Work out the finished part from the listing and answer in its coordinate system (mm). A direction names the side the tool comes from. Give positions to 0.01 mm unless a question says otherwise; leave off trailing zeros. Loops run counter-clockwise (first coordinate to the right, second up) from the corner with the lowest first, then second, coordinate; pieces in that order, holes last. Notation, with made-up numbers: M -21.5,54 L -6.5,54 A22 cw -6.5,92 Z; hole C 55.5,-7 d5. An arc over 180 degrees is marked long. Answer in a Markdown table with one row per item. Add a question column.
from build123d import *

# Parameters (mm, degrees)
BOSS_EXTRUDE1_DEPTH = 1
CUT_EXTRUDE1_DEPTH  = 40.307328833
BOSS_EXTRUDE2_DEPTH = 10
LPATTERN1_COUNT     = 2
LPATTERN1_PITCH     = 20
CUT_EXTRUDE2_REACH  = 73.91
SKETCH4_R           = 1.75
CUT_EXTRUDE3_REACH  = 41.829
SKETCH5_W           = 10
SKETCH5_H           = 6
CHAMFER1_START      = -11.379677933
CHAMFER1_OUTLINE_W  = 13
CHAMFER1_OUTLINE_H  = 2
CHAMFER1_DEPTH      = 16.961310673


with BuildPart() as part:
    # Sketch1 → Boss-Extrude1 (new body)
    with BuildSketch(Plane.XY):
        with BuildLine():
            Line((4.5, -13.81), (34.5, -18.81))
            Line((34.5, -18.81), (34.5, 18.81))
            Line((34.5, 18.81), (-34.5, 18.81))
            Line((-34.5, 18.81), (-34.5, 14.81))
            Line((-34.5, 14.81), (-26.5, 15.18758956))
            ThreePointArc((-26.5, 15.18758956), (-6.254140463, 8.574228065), (4.5, -9.81))
            Line((4.5, -9.81), (4.5, -13.81))
        make_face()
    extrude(amount=BOSS_EXTRUDE1_DEPTH)

    # Sketch2 → Cut-Extrude1 (cut, through all)
    with BuildSketch(Plane.XY.offset(1)):
        with BuildLine():
            Line((7.75, -9.31), (29.75, -9.31))
            ThreePointArc((29.75, -9.31), (31.75, -11.31), (29.75, -13.31))
            Line((29.75, -13.31), (7.75, -13.31))
            ThreePointArc((7.75, -13.31), (5.75, -11.31), (7.75, -9.31))
        make_face()
    extrude(amount=-CUT_EXTRUDE1_DEPTH, mode=Mode.SUBTRACT)

    # Sketch3 → Boss-Extrude2 (add)
    with BuildSketch(Plane(origin=(34.5, 0, 0), x_dir=(0, 0, -1), z_dir=(1, 0, 0))):
        with BuildLine():
            Line((-1, 18.81), (-4.5, 18.81))
            ThreePointArc((-4.5, 18.81), (-7.5, 15.81), (-4.5, 12.81))
            Line((-4.5, 12.81), (-1, 12.81))
            Line((-1, 12.81), (-1, 18.81))
        make_face()
    boss_extrude2 = extrude(amount=-BOSS_EXTRUDE2_DEPTH)

    # LPattern1: Boss-Extrude2 ×2
    with Locations(*[(-i * LPATTERN1_PITCH, 0, 0) for i in range(1, LPATTERN1_COUNT)]):
        add(boss_extrude2)

    # Cut-Extrude2: up to this face of the body (flat: up to its plane)
    cut_extrude2_end = Plane(part.part.faces().sort_by_distance((4.5, 15.81, 3.966377012))[0])
    # Sketch4 → Cut-Extrude2 (cut, up to the picked face)
    with BuildSketch(Plane(origin=(34.5, 0, 0), x_dir=(0, 0, -1), z_dir=(1, 0, 0)), mode=Mode.PRIVATE) as cut_extrude2_sk1:
        with Locations(Location((-4.5, 15.81, 0), (0, 0, 180))):
            Circle(SKETCH4_R)
    cut_extrude2_tool1 = split(extrude(cut_extrude2_sk1.sketch, amount=-CUT_EXTRUDE2_REACH, mode=Mode.PRIVATE), bisect_by=cut_extrude2_end, keep=Keep.BOTH, mode=Mode.PRIVATE)
    add(cut_extrude2_tool1.solids().sort_by(Axis((34.5, 15.81, 4.5), (-1, 0, 0)))[0], mode=Mode.SUBTRACT)

    # Sketch5 → Cut-Extrude3 (cut, up to next)
    with BuildSketch(Plane.XY.offset(1), mode=Mode.PRIVATE) as cut_extrude3_sk1:
        with Locations((19.5, 15.81)):
            Rectangle(SKETCH5_W, SKETCH5_H)
    cut_extrude3_tool1 = extrude(cut_extrude3_sk1.sketch, amount=-CUT_EXTRUDE3_REACH, mode=Mode.PRIVATE) & part.part
    add(cut_extrude3_tool1.solids().sort_by_distance((19.5, 15.81, 1))[0], mode=Mode.SUBTRACT)

    # Chamfer1: read off the stored shape, not the designer's step
    # Chamfer1 outline → Chamfer1 (cut)
    with BuildSketch(Plane(origin=(0, 0, 0), x_dir=(0.937451280255772, -0.34811649938894607, 0), z_dir=(0.34811649938894607, 0.9374512802557721, 0)).offset(CHAMFER1_START)):
        with Locations((-33.5, 0)):
            Rectangle(CHAMFER1_OUTLINE_W, CHAMFER1_OUTLINE_H)
    extrude(amount=CHAMFER1_DEPTH, mode=Mode.SUBTRACT)


solid = part.part
(1) The mould has two halves that part along X. Classify faces 6 (the face through (4.5, 17, 3)), 7 (the face through (15, 4, 1)), 8 (the face through (5.75, -11.35, 0.51)): pulls with the +X half, pulls with the -X half, needs draft (parallel to the pull), parting line crosses it, or undercut.
(2) Section B-B, the plane y = -11.31 is taken. Determine the outline of the cut face in (x, z).
(3) Section A-A, the plane z = 1.75 is taken. Determine the outline of the cut face in (x, y).
(4) Section D-D, the plane x = -14 is taken. Determine the outline of the cut face in (y, z).
(5) Which of the six approach directions +Z, -Z, +X, -X, +Y, -Y give full straight-line access (tool end or side, diameter ignored) to faces 1 (the face through (34.5, 7.1, 0.7)), 2 (the face through (31.75, -11.27, 0.51)), 3 (the face through (30, 12.81, 3)), 4 (the face through (9.6, 15.9, 7.5)), 5 (the face through (14.5, 16, 2))?
(6) Consider line 1 along X through (y, z) = (13.5, 3); line 2 along Z through (x, y) = (30.5, 15.81); line 3 along Y through (x, z) = (7.5, 4.5). Determine where each line is inside the solid, lowest interval first. Write a range as from..to.
(7) Each of these flat-tipped pins is pushed along its axis until it touches: P1, Ø3, axis at y = 15.81, z = 4.5, coming from the -X side; P2, Ø19, axis at x = -4, y = 0, coming from the +Z side; P3, Ø0.5, axis at x = 17.5, z = 0.5, coming from the +Y side; P4, Ø1, axis at x = 32, z = 3.5, coming from the -Y side. Where does it stop, or does it pass through?
(8) Section C-C, the plane z = 5.25 is taken. Determine the outline of the cut face in (x, y).
Numbers:
| question | item | result |
|---|---|---|
| 1 | face 6 | pulls with the -X half |
| 1 | face 7 | needs draft |
| 1 | face 8 | undercut |
| 2 | outline | M 4.5,0 L 5.75,0 L 5.75,1 L 4.5,1 Z; M 31.75,0 L 34.5,0 L 34.5,1 L 31.75,1 Z |
| 3 | outline | M 4.5,12.81 L 14.5,12.81 L 14.5,18.81 L 4.5,18.81 Z; M 24.5,12.81 L 34.5,12.81 L 34.5,18.81 L 24.5,18.81 Z |
| 4 | outline | M 13.1,0 L 18.81,0 L 18.81,1 L 13.1,1 Z |
| 5 | face 1 | +Z, -Z, +X, +Y, -Y |
| 5 | face 2 | +Z, -Z |
| 5 | face 3 | +Z, +X, -X, -Y |
| 5 | face 4 | +Z, +X, -X |
| 5 | face 5 | +Z, -Z, +Y |
| 6 | line 1 | x = 4.5..14.5, 24.5..34.5 |
| 6 | line 2 | z = 0..2.75, 6.25..7.5 |
| 6 | line 3 | y = 12.81..14.06, 17.56..18.81 |
| 7 | P1 | passes through |
| 7 | P2 | stops at z = 1 |
| 7 | P3 | stops at y = 12.81 |
| 7 | P4 | stops at y = 12.81 |
| 8 | outline | M 4.5,12.91 L 14.5,12.91 L 14.5,14.23 L 4.5,14.23 Z; M 4.5,17.39 L 14.5,17.39 L 14.5,18.71 L 4.5,18.71 Z; M 24.5,12.91 L 34.5,12.91 L 34.5,14.23 L 24.5,14.23 Z; M 24.5,17.39 L 34.5,17.39 L 34.5,18.71 L 24.5,18.71 Z |
